Design review of the part shown in the three views and the two pictorial views. Dimensions are in mm from the part's minimum x, y and z. Round coordinates to 2 decimals unless told otherwise and drop trailing zeros. Loops run counter-clockwise (first coordinate to the right, second up) from the corner with the lowest first, then second, coordinate; pieces in that order, holes last.
1. Consider section A-A on z = 25.4. State how many separate pieces and enclosed holes the cut face has, then the cut area to 3 significant figures.
2. To check wall thickness, follow line 1 along Z through (x, y) = (3.5, 38.1); line 2 along Y through (x, z) = (3.5, 25.4); line 3 along Y through (x, z) = (39, 42.5) (1 decimal). State the ranges of each line that lie inside material, in increasing order.
3. Draft analysis for pull direction Y (two halves, no side actions). For the marked faces 1, 2, 3 and 4, state which applies: released by +Y, released by -Y, zero draft, split by the parting line, or undercut.
4. Clearance check with flat-ended pins moving along their axes: pin 1 Ø6 at (y, z) = (44, 15) entering from +X (3 decimals); pin 2 Ø1.5 at (y, z) = (22.5, 32.5) entering from -X; pin 3 Ø4 at (x, z) = (22.5, 8.5) entering from +Y (3 decimals); pin 4 Ø16.5 at (y, z) = (38.1, 25.4) entering from +X. State where each tip first meets the part, or that it passes through.
5. Consider section C-C on x = 24.5. State the section outline as (y, z) points (1 decimal).
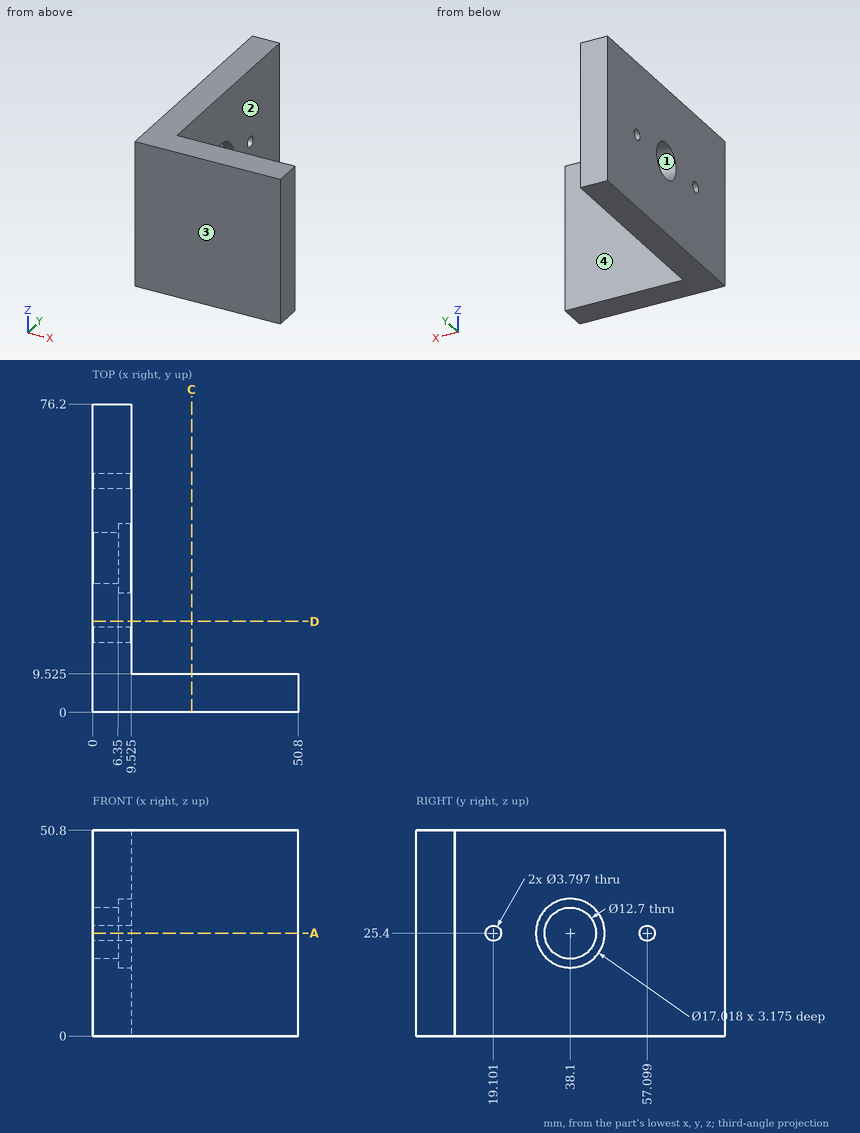
Resolved:
1. separate pieces: 4
1. enclosed holes: 0
1. area: 912 mm2
2. line 1: z = 0 to 19.05, 31.75 to 50.8
2. line 2: y = 0 to 17.2, 21 to 31.75, 44.45 to 55.2, 59 to 76.2
2. line 3: y = 0 to 9.5
3. face 1: undercut
3. face 2: zero draft
3. face 3: released by -Y
3. face 4: released by +Y
4. pin 1: stops at x = 9.525
4. pin 2: stops at x = 0
4. pin 3: stops at y = 9.525
4. pin 4: stops at x = 6.35
5. outline: (0, 0) - (9.5, 0) - (9.5, 50.8) - (0, 50.8) - close
